from build123d import *

# Parameters (mm, degrees)
F0_W      = 108
F0_H      = 140
F1_DEPTH  = 154
F2_R      = 6.5
F3_DEPTH  = 154.001
F4_R      = 16
F5_DEPTH  = 140.001
F6_W      = 108
F6_H      = 55
F7_DEPTH  = 50
F9_DEPTH  = 85.001
F10_W     = 40
F10_H     = 108
F11_DEPTH = 5
F12_R     = 10
F13_DEPTH = 20
F14_R     = 10
F15_DEPTH = 20
F16_W     = 20
F16_H     = 60
F16_W_2   = 44
F16_H_2   = 20
F17_DEPTH = 5
F19_ANGLE = 180


with BuildPart() as f1:
    # F0 (on Right) → F1 (new body)
    with BuildSketch(Plane.YZ):
        Rectangle(F0_W, F0_H)
    extrude(amount=-F1_DEPTH)

    # F2 (on face) → F3 (cut, through all)
    with BuildSketch(Plane(origin=(-154, 0, 0), x_dir=(0, -1, 0), z_dir=(-1, 0, 0))):
        with Locations((-42, 47)):
            Circle(F2_R)
        with Locations((42, 47)):
            Circle(F2_R)
        with Locations((-42, -47)):
            Circle(F2_R)
        with Locations((42, -47)):
            Circle(F2_R)
    extrude(amount=-F3_DEPTH, mode=Mode.SUBTRACT)

    # F4 (on face) → F5 (cut, through all)
    with BuildSketch(Plane(origin=(0, 0, -70), x_dir=(1, 0, 0), z_dir=(0, 0, -1))):
        with Locations((-125, 0)):
            Circle(F4_R)
        with Locations((-80, 0)):
            Circle(F4_R)
    extrude(amount=-F5_DEPTH, mode=Mode.SUBTRACT)

    # F6 (on face) → F7 (cut)
    with BuildSketch(Plane(origin=(-154, 0, 0), x_dir=(0, -1, 0), z_dir=(-1, 0, 0))):
        with Locations((0, -42.5)):
            Rectangle(F6_W, F6_H)
    extrude(amount=-F7_DEPTH, mode=Mode.SUBTRACT)

    # F8 (on face) → F9 (cut, through all)
    with BuildSketch(Plane(origin=(0, 0, -15), x_dir=(1, 0, 0), z_dir=(0, 0, -1))):
        Polygon((-154, -54), (-119, -54), (-119, -30), (-141.0096189432, -30), (-154, -22.5), align=None)
        Polygon((-119, 30), (-119, 54), (-154, 54), (-154, 22.5), (-141.0096189432, 30), align=None)
    extrude(amount=-F9_DEPTH, mode=Mode.SUBTRACT)

    # F10 (on face) → F11 (cut)
    with BuildSketch(Plane(origin=(0, 0, -70), x_dir=(1, 0, 0), z_dir=(0, 0, -1))):
        with Locations((-20, 0)):
            Rectangle(F10_W, F10_H)
    extrude(amount=-F11_DEPTH, mode=Mode.SUBTRACT)

    # F12 (on face) → F13 (cut)
    with BuildSketch(Plane(origin=(-104, 0, 0), x_dir=(0, -1, 0), z_dir=(-1, 0, 0))):
        with Locations((-42, -47)):
            Circle(F12_R)
        with Locations((42, -47)):
            Circle(F12_R)
    extrude(amount=-F13_DEPTH, mode=Mode.SUBTRACT)

    # F14 (on face) → F15 (cut)
    with BuildSketch(Plane(origin=(-119, 0, 0), x_dir=(0, -1, 0), z_dir=(-1, 0, 0))):
        with Locations((-42, 47)):
            Circle(F14_R)
        with Locations((42, 47)):
            Circle(F14_R)
    extrude(amount=-F15_DEPTH, mode=Mode.SUBTRACT)

    # F16 (on face) → F17 (cut)
    with BuildSketch(Plane.YZ):
        with Locations((0, 40)):
            Rectangle(F16_W, F16_H)
        with Locations((32, 0)):
            Rectangle(F16_W_2, F16_H_2)
        Rectangle(F16_W, F16_H_2)
        with Locations((-32, 0)):
            Rectangle(F16_W_2, F16_H_2)
        with Locations((0, -40)):
            Rectangle(F16_W, F16_H)
    extrude(amount=-F17_DEPTH, mode=Mode.SUBTRACT)


with BuildPart() as f1_1:
    # F19: moved
    add(f1.part.rotate(Axis((58.3656840026, 0, 0), (1, 0, 0)), F19_ANGLE))


solid = f1_1.part
Verification items for the finished model (mm, model axes). A direction names the side the tool comes from. Round coordinates to 2 decimals unless told otherwise and drop trailing zeros. Loops run counter-clockwise (first coordinate to the right, second up) from the corner with the lowest first, then second, coordinate; pieces in that order, holes last. Notation, with made-up numbers: (47, 31) - (60, 31) arc R17 cw to (60, 56) - close; hole circle Ø8 at (74, 24.5). An arc over 180 degrees is marked (long way). Use one line per item in the form item = value.
1. Scan lines: probe 1 along Z at (x, y) = (-62, -42); probe 2 along Z at (x, y) = (-38, -42); probe 3 along Y at (x, z) = (-45, 42.5). Record each from-to range of solid material in increasing order.
A:
probe_1 = -70 to -53.5, -40.5 to 40.5, 53.5 to 70
probe_2 = -70 to -53.5, -40.5 to 40.5, 53.5 to 65
probe_3 = -54 to -46.69, -37.31 to 37.31, 46.69 to 54
2. Section check D-D on x = -59. Record the cut outline in (y, z).
A:
outline = (-54, -70) - (54, -70) - (54, 70) - (-54, 70) - close; hole circle Ø13 at (-42, -47); hole circle Ø13 at (-42, 47); hole circle Ø13 at (42, -47); hole circle Ø13 at (42, 47)
3. Draft check along Y on faces 5 (the flat face through (-119, 42, -27)), 6 (the flat face through (-130, -30, -27)), 7 (the cylindrical face through (-94.14, -44.17, 56.76)), 8 (the flat face through (-84, 42, 54)). Enter one of: pulls with the +Y half, pulls with the -Y half, needs draft (parallel to the pull), parting line crosses it, or undercut.
A:
face_5 = needs draft
face_6 = pulls with the -Y half
face_7 = undercut
face_8 = undercut
4. Section check A-A on z = 47. Record the cut outline in (x, y), and give its area (3 significant figures).
A:
outline = (-104, -54) - (0, -54) - (0, -48.5) - (-84, -48.5) - (-84, -52) - (-104, -52) - close; (-104, -32) - (-84, -32) - (-84, -35.5) - (0, -35.5) - (0, -10) - (-5, -10) - (-5, 10) - (0, 10) - (0, 35.5) - (-84, 35.5) - (-84, 32) - (-104, 32) - close; (-104, 52) - (-84, 52) - (-84, 48.5) - (0, 48.5) - (0, 54) - (-104, 54) - close; hole circle Ø32 at (-80, 0)
area = 7,340 mm²
5. Section check C-C on y = 0. Record the cut outline in (x, z), and give its area (3 significant figures).
A:
outline = (-154, -70) - (-141, -70) - (-141, 15) - (-154, 15) - close; (-109, -70) - (-96, -70) - (-96, 70) - (-104, 70) - (-104, 15) - (-109, 15) - close; (-64, -70) - (-5, -70) - (-5, 65) - (-40, 65) - (-40, 70) - (-64, 70) - close
area = 10,700 mm²
6. Gauge pin test, flat ends, axial feed: pin 1 Ø12 at (y, z) = (44, -7) entering from -X; pin 2 Ø12 at (x, y) = (-29, -1.5) entering from +Z; pin 3 Ø1.5 at (y, z) = (2, 66.5) entering from +X; pin 4 Ø11.5 at (y, z) = (-42, 47) entering from +X. Record the tip position at first contact, or that the pin passes through.
A:
pin_1 = -119
pin_2 = 65
pin_3 = -40
pin_4 = through
7. Access from +Z, -Z, +X, -X, +Y, -Y to the whole of each face (thin tool, end or side, straight path). Record for faces 1 (the cylindrical face through (-109.14, -44.17, -37.24)), 2 (the flat face through (-104, -1, 42)), 3 (the flat face through (-2, 32, -10)), 4 (the flat face through (-2, 10, 38)).
A:
face_1 = -X
face_2 = +Z, -X, +Y, -Y
face_3 = +X, +Y, -Y
face_4 = +Z, -Z, +X
8. Section check B-B on x = -80. Record the cut outline in (y, z), and give its area (3 significant figures).
A:
outline = (-54, -70) - (-16, -70) - (-16, 70) - (-54, 70) - close; (16, -70) - (54, -70) - (54, 70) - (16, 70) - close; hole circle Ø13 at (-42, -47); hole circle Ø13 at (-42, 47); hole circle Ø13 at (42, -47); hole circle Ø13 at (42, 47)
area = 10,100 mm²
